Work out the finished part from the listing and answer in its coordinate system (mm). Face numbers are marked on the shaded views. A direction names the side the tool comes from. Give positions to 0.01 mm unless a question says otherwise; leave off trailing zeros. Order: outer loops, then holes, each group sorted by start corner. A loop starts at its lowest first (then second) coordinate and runs counter-clockwise, first axis right, second up. Notation, with made-up numbers: (14.25, -20) - (72.25, -20) arc R32 ccw to (72.25, 10) - close; hole circle Ø1 at (56.25, -36.5). An arc over 180 degrees is marked (long way). Write each question's results on one line, items separated by ' | '.
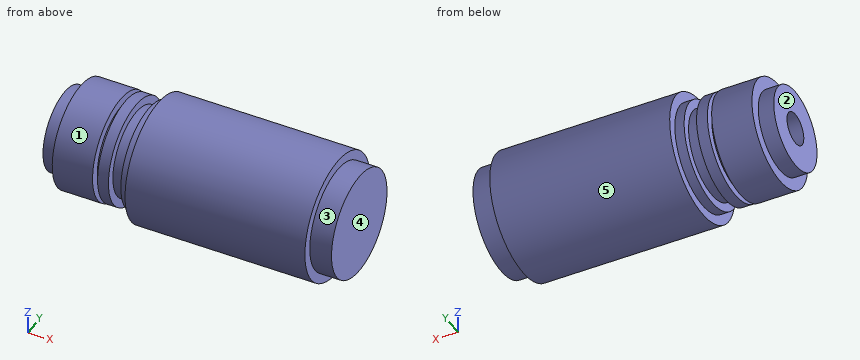
from build123d import *

# Parameters (mm, degrees)
F3_D     = 10.3
F3_DEPTH = 17.25
F3_TIP   = 3.094432188


with BuildPart() as f1:
    # F0 (on Front) → F1 (revolve)
    with BuildSketch(Plane.XZ):
        Polygon((-66.909504354, 13.3051262531), (-66.909504354, 0.0551262531), (28.090495646, 0.0551262531), (28.090495646, 17.0551262531), (21.090495646, 17.0551262531), (21.090495646, 20.0551262531), (-36.909504354, 20.0551262531), (-36.909504354, 16.9051262531), (-39.909504354, 16.9051262531), (-39.909504354, 14.2051262531), (-43.909504354, 14.2051262531), (-43.909504354, 16.9051262531), (-47.409504354, 16.9051262531), (-47.409504354, 14.2051262531), (-48.909504354, 14.2051262531), (-48.909504354, 17.1507116718), (-61.909504354, 17.1507116718), (-61.909504354, 13.3051262531), align=None)
    revolve(axis=Axis((-19.409504354, 0, 0.0551262531), (1, 0, 0)))

    # F3
    with Locations(Plane(origin=(-66.909504354, 0, 0), x_dir=(0, -1, 0), z_dir=(-1, 0, 0))):
        with Locations((0, 0)):
            Hole(F3_D / 2, depth=F3_DEPTH)
            with Locations((0, 0, -(F3_DEPTH + F3_TIP / 2))):  # 118° drill point
                Cone(0, F3_D / 2, F3_TIP, mode=Mode.SUBTRACT)


solid = f1.part
1. Determine the mould class of the marked faces 4 and 5 for opening direction Y: +Y half, -Y half, draft (parallel to the pull), parting line (faces both ways), or undercut.
Answer list:
face 4: draft | face 5: parting line
2. A tool of negligible diameter and unlimited length cuts with its end or side. For the marked faces 1, 2 and 3, from which of +Z, -Z, +X, -X, +Y, -Y can it reach the whole face along a straight path? Write none if from no direction.
Answer list:
face 1: -X | face 2: +Z, -Z, -X, +Y, -Y | face 3: +X
3. A cutting plane is placed at D-D, the plane x = 22. Write down the section's boundary in (y, z).
Answer list:
outline: circle Ø34 at (0, 0.06)
4. A cutting plane is placed at B-B, the plane x = -60. Write down the section's boundary in (y, z), then the cut area to 3 significant figures.
Answer list:
outline: circle Ø34.19 at (0, 0.06); hole circle Ø10.3 at (0, 0) | area: 835 mm^2
5. Given P1, Ø6, axis at x = -11.5, y = 12.5, coming from the -Z side; P2, Ø5, axis at x = -31, y = -16, coming from the -Z side; P3, Ø1.5, axis at x = -29.5, y = 5, coming from the -Z side, each flat-ended and moving along its own axis, determine where each tip first touches the part or whether it passes through.
Answer list:
P1: z = -17.54 | P2: z = -14.7 | P3: z = -19.49
6. Straight lines are drawn through the part: line 1 (X direction, y = -2, z = -14); line 2 (Z direction, x = -58.5, y = 0); line 3 (Y direction, x = -58.5, z = 0). For each, find the intervals that lie inside material, in ascending order. Write a range as [from, to].
Answer list:
line 1: [-61.91, -48.91], [-47.41, -43.91], [-39.91, 28.09] | line 2: [-17.04, -5.15], [5.15, 17.15] | line 3: [-17.1, -5.15], [5.15, 17.1]
